```python
from build123d import *

# Parameters (mm, degrees)
SKETCH1_W              = 254
SKETCH1_H              = 101.6
BOSS_EXTRUDE1_DEPTH    = 3.175
F_4_CLEARANCE_HOLE1_D  = 3.2639
F_10_CLEARANCE_HOLE1_D = 5.1054


with BuildPart() as part:
    # Sketch1 → Boss-Extrude1 (new, symmetric)
    with BuildSketch(Plane.XY):
        Rectangle(SKETCH1_W, SKETCH1_H)
    extrude(amount=BOSS_EXTRUDE1_DEPTH, both=True)

    # #4 Clearance Hole1 (through all)
    with Locations(Plane.XY.offset(3.175)):
        with Locations((-120.65, 47.625), (-120.65, 28.575), (-120.65, 9.525), (-120.65, -9.525), (-120.65, -28.575), (-120.65, -47.625)):
            f_4_clearance_hole1 = Hole(F_4_CLEARANCE_HOLE1_D / 2)

    # Mirror1: #4 Clearance Hole1 across plane
    add(f_4_clearance_hole1.mirror(Plane(origin=(0, 0, 0), x_dir=(0, 0, 1), z_dir=(1, 0, 0))), mode=Mode.SUBTRACT)

    # #10 Clearance Hole1 (through all)
    with Locations(Plane.XY.offset(3.175)):
        with Locations((-24.659484021, 12.7), (26.140515979, 12.7), (26.140515979, -12.7), (-24.659484021, -12.7)):
            Hole(F_10_CLEARANCE_HOLE1_D / 2)


solid = part.part
```
Here's how the part is built. I have some questions about the finished solid (model axes, mm). Give positions to 0.01 mm unless a question says otherwise; leave off trailing zeros. Put each result on its own line as item: value. Start each with the question number.
Item 1: I need wall thicknesses on L1, parallel to X at y = 9.5, z = -0.5; L2, parallel to X at y = 27.5, z = -1.25; L3, parallel to X at y = -10.5, z = -2.5. Which ranges of each line are inside material? Lowest first, please. Write a range as from..to.
Item 2: Will this pin go through, and if not, where does the flat tip stop? pin 1 (2.5 mm diameter, centred on x = 120.65, y = -28.575, fed in from +Z).
Item 3: Thinking about a two-plate mould opening in Y: for faces 1 (the cylindrical face through (-27.018, -13.678, -0.044)), 2 (the cylindrical face through (-27.018, 11.722, -0.044)), 3 (the flat face through (-2, -50.8, 0)), 4 (the flat face through (-127, -1, 0)), which applies, +Y half, -Y half, draft (parallel to the pull), parting line (faces both ways), or undercut?
Values:
1. L1: -127..-122.28, -119.02..119.02, 122.28..127
1. L2: -127..-121.88, -119.42..119.42, 121.88..127
1. L3: -127..-121.96, -119.34..-25.95, -23.36..24.85, 27.44..119.34, 121.96..127
2. pin 1: through
3. face 1: undercut
3. face 2: undercut
3. face 3: -Y half
3. face 4: draft
